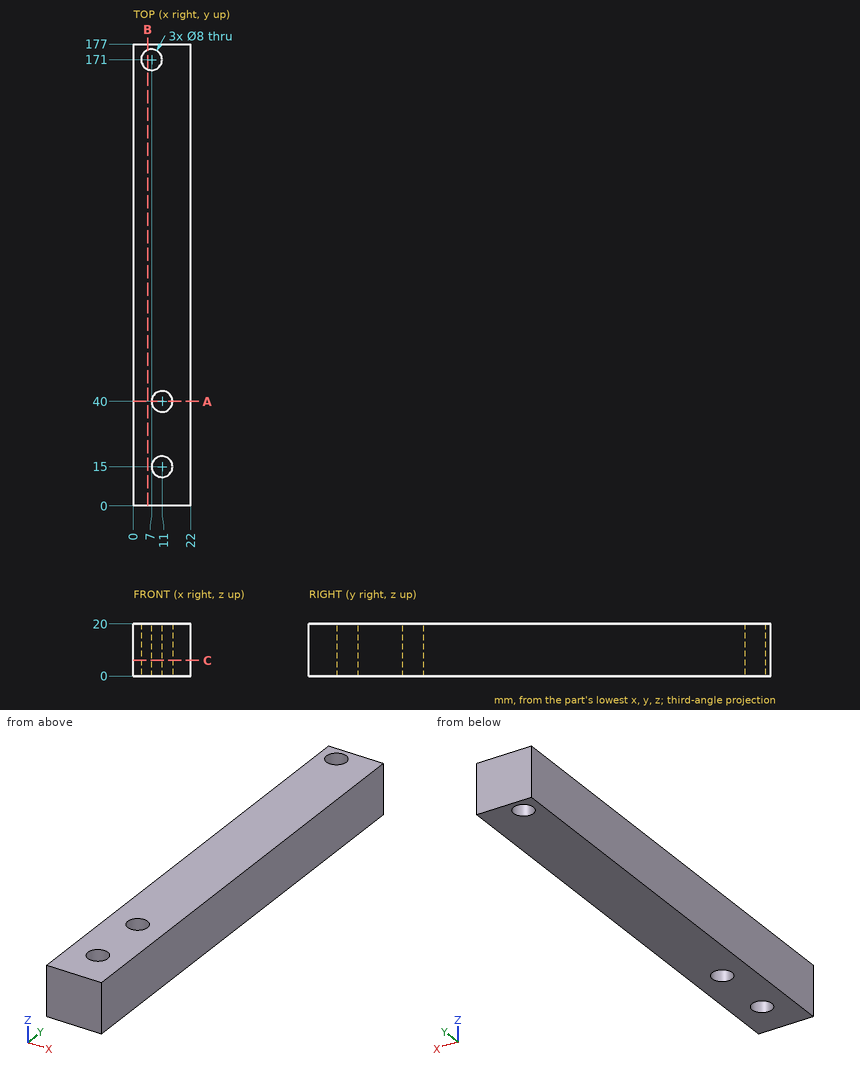
Source: three-view drawing plus pictorial views. Frame: mm from the lowest corner of the part. Give positions to 0.01 mm unless a question says otherwise; leave off trailing zeros. Loops run counter-clockwise (first coordinate to the right, second up) from the corner with the lowest first, then second, coordinate; pieces in that order, holes last. Notation, with made-up numbers: (-23.75, -15.5) -> (-19.75, -15.5) arc R21 cw to (-19.75, -8.5) -> close; hole circle Ø8 at (46, 81.5). An arc over 180 degrees is marked (long way). Put each result on its own line as item: value. Start each with the question number.
1) Cut plane C-C (z = 6). Return loops of the section in (x, y), then the cut area to 3 significant figures.
2) Cut plane A-A (y = 40). Return loops of the section in (x, z), then the cut area to 3 significant figures.
3) Material intervals for probe 1 along Y at (x, z) = (11.5, 12.5); probe 2 along Y at (x, z) = (8.5, 19); probe 3 along X at (y, z) = (41.5, 10.5), sorted ascending.
4) Cut plane B-B (x = 5.5). Return loops of the section in (y, z), then the cut area to 3 significant figures.
Results are:
1. outline: (0, 0) -> (22, 0) -> (22, 177) -> (0, 177) -> close; hole circle Ø8 at (7, 171); hole circle Ø8 at (11, 15); hole circle Ø8 at (11, 40)
1. area: 3,740 mm2
2. outline: (0, 0) -> (7, 0) -> (7, 20) -> (0, 20) -> close; (15, 0) -> (22, 0) -> (22, 20) -> (15, 20) -> close
2. area: 280 mm2
3. probe 1: y = 0 to 11.03, 18.97 to 36.03, 43.97 to 177
3. probe 2: y = 0 to 11.88, 18.12 to 36.88, 43.12 to 167.29, 174.71 to 177
3. probe 3: x = 0 to 7.29, 14.71 to 22
4. outline: (0, 0) -> (167.29, 0) -> (167.29, 20) -> (0, 20) -> close; (174.71, 0) -> (177, 0) -> (177, 20) -> (174.71, 20) -> close
4. area: 3,390 mm2
